Source: CAD feature listing. Evaluate the final solid. Frame: model axes, mm. Face numbers are marked on the shaded views. A direction names the side the tool comes from. Round coordinates to 2 decimals unless told otherwise and drop trailing zeros. Write each loop counter-clockwise with the first axis right and the second up, starting at its lowest first coordinate (ties: lowest second). Pieces come first, ordered by that corner, then holes. Notation, with made-up numbers: M 23.25,-27 L 65.25,-27 A27 ccw 65.25,4 Z; hole C 69,80.5 d7. An arc over 180 degrees is marked long. Answer in a Markdown table with one row per item. Add a question column.
Item 1: Cut plane D-D on y = 5.75. Return loops of the section in (x, z), and give its area (3 significant figures).
Item 2: Set-up query: the marked faces 5 and 6. Return all of +Z, -Z, +X, -X, +Y, -Y with unobstructed straight access to the full face (end or side cutting, diameter ignored); none if empty.
Item 3: Material intervals for probe 1 along X at (y, z) = (7.3, 0); probe 2 along Z at (x, y) = (0, 3.5); probe 3 along Y at (x, z) = (-5.5, 1.5), sorted ascending.
Item 4: Cut plane A-A on y = 3. Return loops of the section in (x, z), and give its area (3 significant figures).
Item 5: Contact query for flat-ended pins moving along their axis: pin 1 (2 mm diameter, centred on x = 2.5, z = -0.5, fed in from +Y); pin 2 (6.5 mm diameter, centred on x = 0, z = 0, fed in from -Y). Output: stop coordinate, or through.
Item 6: Cut plane C-C on x = -3.25. Return loops of the section in (y, z).
Item 7: Cut plane B-B on z = -1.25. Return loops of the section in (x, y).
Item 8: Mould query, pull axis Z, two halves, no side actions, for the marked faces 1, 2, 3 and 4. Classes: released by +Z, released by -Z, zero draft, split by the parting line, or undercut.
from build123d import *

# Parameters (mm, degrees)
SKETCH1_R           = 3.45
BOSS_EXTRUDE1_DEPTH = 8
SKETCH2_R           = 4.05
CUT_EXTRUDE1_DEPTH  = 3
SKETCH3_R           = 10
SKETCH3_R_2         = 5.5
CUT_EXTRUDE3_DEPTH  = 4


with BuildPart() as part:
    # Sketch1 → Boss-Extrude1 (new body)
    with BuildSketch(Plane(origin=(0, 0, 0), x_dir=(1, 0, 0), z_dir=(0, 1, 0))):
        Polygon((3.464101615, 6), (-3.464101615, 6), (-6.92820323, 0), (-3.464101615, -6), (3.464101615, -6), (6.92820323, 0), align=None)
        Circle(SKETCH1_R, mode=Mode.SUBTRACT)
    extrude(amount=BOSS_EXTRUDE1_DEPTH)

    # Sketch2 → Cut-Extrude1 (cut)
    with BuildSketch(Plane(origin=(0, 8, 0), x_dir=(1, 0, 0), z_dir=(0, 1, 0))):
        Circle(SKETCH2_R)
    extrude(amount=-CUT_EXTRUDE1_DEPTH, mode=Mode.SUBTRACT)

    # Sketch3 → Cut-Extrude3 (cut)
    with BuildSketch(Plane(origin=(0, 8, 0), x_dir=(1, 0, 0), z_dir=(0, 1, 0))):
        Circle(SKETCH3_R)
        Polygon((6.92820323, 0), (3.464101615, 6), (-3.464101615, 6), (-6.92820323, 0), (-3.464101615, -6), (3.464101615, -6), align=None, mode=Mode.SUBTRACT)
        Polygon((3.464101615, -6), (6.92820323, 0), (3.464101615, 6), (-3.464101615, 6), (-6.92820323, 0), (-3.464101615, -6), align=None)
        Circle(SKETCH3_R_2, mode=Mode.SUBTRACT)
    extrude(amount=-CUT_EXTRUDE3_DEPTH, mode=Mode.SUBTRACT)


solid = part.part
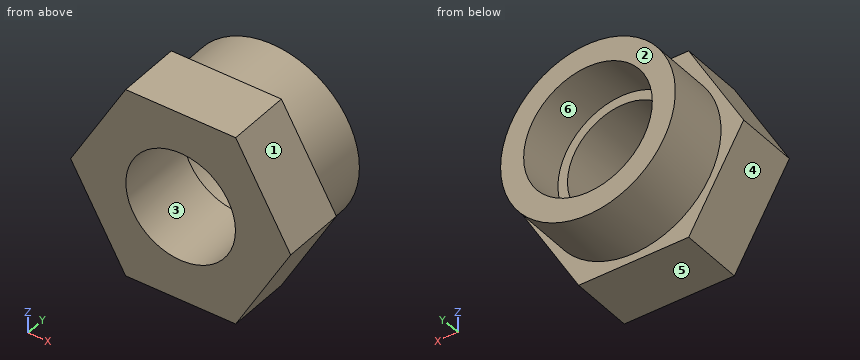
Results below:
| question | item | result |
|---|---|---|
| 1 | outline | C 0,0 d11; hole C 0,0 d8.1 |
| 1 | area | 43.5 mm2 |
| 2 | face 5 | -Z, +X, -X, +Y, -Y |
| 2 | face 6 | +Y |
| 3 | probe 1 | -5.5 to -4.05, 4.05 to 5.5 |
| 3 | probe 2 | -6 to -3.45, 3.45 to 6 |
| 3 | probe 3 | 0 to 4 |
| 4 | outline | M -6.93,0 L -3.46,-6 L 3.46,-6 L 6.93,0 L 3.46,6 L -3.46,6 Z; hole C 0,0 d6.9 |
| 4 | area | 87.3 mm2 |
| 5 | pin 1 | y = 5 |
| 5 | pin 2 | through |
| 6 | outline | M 0,-6 L 4,-6 L 4,-4.44 L 8,-4.44 L 8,-2.42 L 5,-2.42 L 5,-1.16 L 0,-1.16 Z; M 0,1.16 L 5,1.16 L 5,2.42 L 8,2.42 L 8,4.44 L 4,4.44 L 4,6 L 0,6 Z |
| 7 | outline | M -6.21,0 L -3.22,0 L -3.22,5 L -3.85,5 L -3.85,8 L -5.36,8 L -5.36,4 L -6.21,4 Z; M 3.22,0 L 6.21,0 L 6.21,4 L 5.36,4 L 5.36,8 L 3.85,8 L 3.85,5 L 3.22,5 Z |
| 8 | face 1 | released by +Z |
| 8 | face 2 | zero draft |
| 8 | face 3 | undercut |
| 8 | face 4 | released by -Z |
